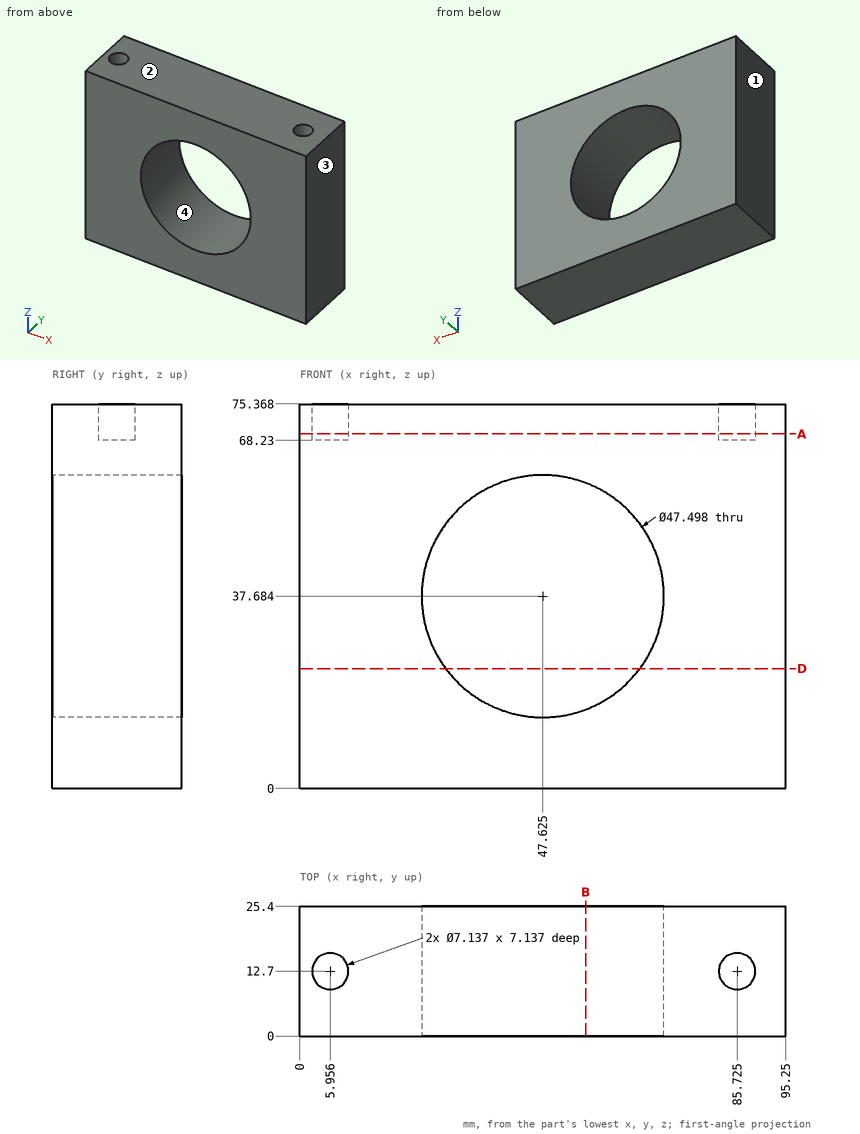
Design review of the part shown in the three views and the two pictorial views. Dimensions are in mm from the part's minimum x, y and z. Coordinates: 2 decimals unless noted, no trailing zeros. Write each loop counter-clockwise with the first axis right and the second up, starting at its lowest first coordinate (ties: lowest second). Pieces come first, ordered by that corner, then holes.
(1) The part is to be moulded in two halves that separate along X. For the marked faces 1, 2, 3 and 4, say which applies: +X half, -X half, draft (parallel to the pull), parting line (faces both ways), or undercut.
(2) For pin 1 Ø3.5 at (x, y) = (4.5, 12.5) entering from +Z, flat-tipped, find the tip position at first contact; note if it passes through.
(3) Add section B-B on x = 56. Give the boundary of the cut face in (y, z).
(4) Add section A-A on z = 69.5. Count the separate pieces of the cut face and the enclosed holes in it, then the cut area to 3 significant figures.
(5) Wall thickness on probe 1 along Z at (x, y) = (9, 12); probe 2 along X at (y, z) = (13, 40); probe 3 along X at (y, z) = (11.25, 22): over which ranges is each line inside the solid? List them lowest first.
(6) Add section D-D on z = 23.5. Give the boundary of the cut face in (x, y).
Answer sheet:
1. face 1: -X half
1. face 2: draft
1. face 3: +X half
1. face 4: undercut
2. pin 1: stops at z = 68.23
3. outline: (0, 0) - (25.4, 0) - (25.4, 15.46) - (0, 15.46) - close; (0, 59.91) - (25.4, 59.91) - (25.4, 75.37) - (0, 75.37) - close
4. separate pieces: 1
4. enclosed holes: 2
4. area: 2,340 mm2
5. probe 1: z = 0 to 68.23
5. probe 2: x = 0 to 23.99, 71.26 to 95.25
5. probe 3: x = 0 to 29.79, 65.46 to 95.25
6. outline: (0, 0) - (28.58, 0) - (28.58, 25.4) - (0, 25.4) - close; (66.67, 0) - (95.25, 0) - (95.25, 25.4) - (66.67, 25.4) - close
